from build123d import *

# Parameters (mm, degrees)
F1_E1_W  = 76.2
F1_E1_H  = 3.9751
F3_E0_W  = 76.2
F3_E0_H  = 3.9751
F5_E3_W  = 108.4099765605
F5_E3_H  = 3.9751
F7_E2_W  = 108.4099765605
F7_E2_H  = 3.9751
F9_E4_W  = 77.1121457219
F9_E4_H  = 3.9751
F11_E5_W = 145.6045582891
F11_E5_H = 3.9751


with BuildPart() as f2:
    # F1_E1 (on explicit) → F2 (revolve)
    with BuildSketch(Plane(origin=(0, 0, 0), x_dir=(-1, 0, 0), z_dir=(0, 1, 0))):
        with Locations((38.1, 1.98755)):
            Rectangle(F1_E1_W, F1_E1_H)
    revolve(axis=Axis((-38.1, 0, 0), (-1, 0, 0)))

    # F3_E0 (on explicit) → F4 (revolve)
    with BuildSketch(Plane.XZ):
        with Locations((38.1, 1.98755)):
            Rectangle(F3_E0_W, F3_E0_H)
    revolve(axis=Axis((38.1, 0, 0), (1, 0, 0)))

    # F5_E3 (on explicit) → F6 (revolve)
    with BuildSketch(Plane(origin=(0, -77.1121457219, 0), x_dir=(0.7028873395, 0.7113011936, 0), z_dir=(0.7113011936, -0.7028873395, 0))):
        with Locations((54.2049882802, 1.98755)):
            Rectangle(F5_E3_W, F5_E3_H)
    revolve(axis=Axis((38.1, -38.556072861, 0), (0.7028873395, 0.7113011936, 0)))

    # F7_E2 (on explicit) → F8 (revolve)
    with BuildSketch(Plane(origin=(-76.2, 0, 0), x_dir=(0.7028873395, -0.7113011936, 0), z_dir=(-0.7113011936, -0.7028873395, 0))):
        with Locations((54.2049882802, 1.98755)):
            Rectangle(F7_E2_W, F7_E2_H)
    revolve(axis=Axis((-38.1, -38.556072861, 0), (0.7028873395, -0.7113011936, 0)))

    # F9_E4 (on explicit) → F10 (revolve)
    with BuildSketch(Plane(origin=(0, 0, 0), x_dir=(0, -1, 0), z_dir=(-1, 0, 0))):
        with Locations((38.556072861, 1.98755)):
            Rectangle(F9_E4_W, F9_E4_H)
    revolve(axis=Axis((0, -38.556072861, 0), (0, -1, 0)))

    # F11_E5 (on explicit) → F12 (revolve)
    with BuildSketch(Plane(origin=(0, -77.1121457219, 0), x_dir=(0, -1, 0), z_dir=(-1, 0, 0))):
        with Locations((72.8022791445, 1.98755)):
            Rectangle(F11_E5_W, F11_E5_H)
    revolve(axis=Axis((0, -149.9144248664, 0), (0, -1, 0)))


solid = f2.part
Could you check a few things on this model? Use its own coordinates, in mm. Give positions to 0.01 mm unless a question says otherwise; leave off trailing zeros. Order: outer loops, then holes, each group sorted by start corner. A loop starts at its lowest first (then second) coordinate and runs counter-clockwise, first axis right, second up. Notation, with made-up numbers: (43, -27.75) - (55, -27.75) arc R9 cw to (55, -23.75) - close; hole circle Ø9 at (36, 61). An arc over 180 degrees is marked (long way). One line per item, written item: value. Start each with the question number.
1. Imagine slicing it at A-A on z = 0. List the corners of the cut face in (x, y) for me, plus the area to 3 significant figures.
2. For P1, Ø1.2, axis at y = 1, z = 1.5, coming from the -X side; P2, Ø4, axis at x = 24, z = -2.5, coming from the -Y side; P3, Ø1.2, axis at y = 1, z = 2, coming from the +X side, each with a flat end and sliding along its axis, tell me the tip position at first contact or that it passes through.
3. If I drill on probe 1 along Y at (x, z) = (-21, -1.25); probe 2 along Y at (x, z) = (-32.5, -1.25); probe 3 along X at (y, z) = (-136.5, 1.5), over which ranges is the centre line in solid material (lowest first)?
4. Imagine slicing it at B-B on y = -132.5. List the corners of the cut face in (x, z) for me.
5. Thinking about a two-plate mould opening in X: for faces 1 (the face through (0, -222.717, 0)), 2 (the face through (1.522, -150.934, 3.672)), 3 (the face through (1.07, 3.88, -0.86)), which applies, +X half, -X half, draft (parallel to the pull), parting line (faces both ways), or undercut?
Values:
1. outline: (-79.03, -2.79) - (-3.98, -78.74) - (-3.98, -222.72) - (3.98, -222.72) - (3.98, -78.74) - (79.03, -2.79) - (76.2, 0) - (76.2, 3.98) - (-76.2, 3.98) - (-76.2, 0) - close; hole (-66.68, -3.98) - (-3.98, -67.43) - (-3.98, -3.98) - close; hole (3.98, -67.43) - (66.68, -3.98) - (3.98, -3.98) - close
1. area: 4,510 mm²
2. P1: x = -76.2
2. P2: y = -59.81
2. P3: x = 76.2
3. probe 1: -61.23 to -50.49, -3.77 to 3.77
3. probe 2: -49.59 to -38.85, -3.77 to 3.77
3. probe 3: -3.68 to 3.68
4. outline: circle Ø7.95 at (0, 0)
5. face 1: draft
5. face 2: parting line
5. face 3: undercut
